Geometry check sheet. Reference: the model listing, model coordinates, mm. Give positions to 0.01 mm unless a question says otherwise; leave off trailing zeros. Order: outer loops, then holes, each group sorted by start corner. A loop starts at its lowest first (then second) coordinate and runs counter-clockwise, first axis right, second up. Notation, with made-up numbers: M 37.25,74 L 92.25,74 A16 ccw 92.25,91 Z; hole C -14.75,-38.5 d11. An arc over 180 degrees is marked long. Put each result on its own line as item: value. Start each with the question number.
Q1. Go/stop test with a flat-tipped pin: pin 1 (6 mm diameter, centred on x = 12, y = -4.5, fed in from +Z). Record where the tip stops, or that it passes through.
Q2. Section check C-C on z = 0.65. Record the cut outline in (x, y).
Q3. Material ranges on L1, parallel to Y at x = -2.5, z = 2.65; L2, parallel to X at y = -2.5, z = 1.1; L3, parallel to Y at x = -20, z = 1.2, recorded low to high.
Q4. Section check A-A on y = 0. Record the cut outline in (x, z), then the cut area to 3 significant figures.
Q5. Section check D-D on x = -4.5. Record the cut outline in (y, z).
Q6. Section check B-B on x = 20. Record the cut outline in (y, z), then the cut area to 3 significant figures.
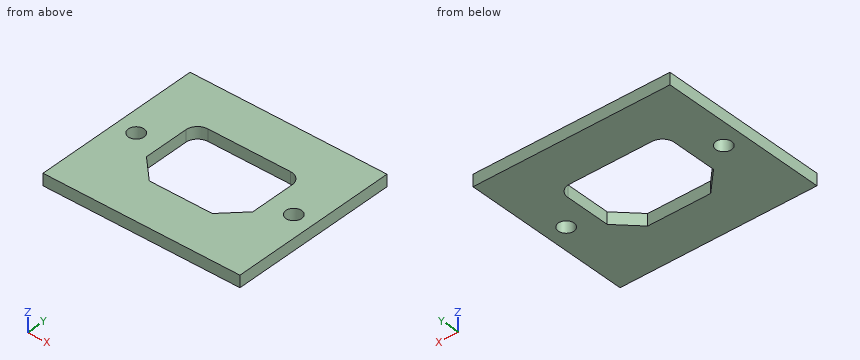
```python
from build123d import *

# Parameters (mm, degrees)
F0_W     = 50
F0_H     = 43
F0_R     = 2
F0_W_2   = 27
F0_H_2   = 20
F1_DEPTH = 3
F2_R     = 3
F3_SIZE  = 5.5


with BuildPart() as f1:
    # F0 (on Top) → F1 (new body)
    with BuildSketch(Plane.XY):
        Rectangle(F0_W, F0_H)
        with Locations((-20, 0)):
            Circle(F0_R, mode=Mode.SUBTRACT)
        Rectangle(F0_W_2, F0_H_2, mode=Mode.SUBTRACT)
        with Locations((20, 0)):
            Circle(F0_R, mode=Mode.SUBTRACT)
    extrude(amount=F1_DEPTH)

    # F2
    f2_edges = [f1.edges().sort_by_distance(p)[0] for p in [
        (-13.5, 10, 1.5),
        (13.5, 10, 1.5),
    ]]
    fillet(f2_edges, radius=F2_R)

    # F3
    f3_edges = [f1.edges().sort_by_distance(p)[0] for p in [
        (-13.5, -10, 1.5),
        (13.5, -10, 1.5),
    ]]
    chamfer(f3_edges, length=F3_SIZE)


solid = f1.part
```
Results found:
1. pin 1: stops at z = 3
2. outline: M -25,-21.5 L 25,-21.5 L 25,21.5 L -25,21.5 Z; hole C -20,0 d4; hole M -13.5,-4.5 L -8,-10 L 8,-10 L 13.5,-4.5 L 13.5,7 A3 ccw 10.5,10 L -10.5,10 A3 ccw -13.5,7 Z; hole C 20,0 d4
3. L1: y = -21.5 to -10, 10 to 21.5
3. L2: x = -25 to -13.5, 13.5 to 25
3. L3: y = -21.5 to -2, 2 to 21.5
4. outline: M -25,0 L -22,0 L -22,3 L -25,3 Z; M -18,0 L -13.5,0 L -13.5,3 L -18,3 Z; M 13.5,0 L 18,0 L 18,3 L 13.5,3 Z; M 22,0 L 25,0 L 25,3 L 22,3 Z
4. area: 45.0 mm^2
5. outline: M -21.5,0 L -10,0 L -10,3 L -21.5,3 Z; M 10,0 L 21.5,0 L 21.5,3 L 10,3 Z
6. outline: M -21.5,0 L -2,0 L -2,3 L -21.5,3 Z; M 2,0 L 21.5,0 L 21.5,3 L 2,3 Z
6. area: 117 mm^2
